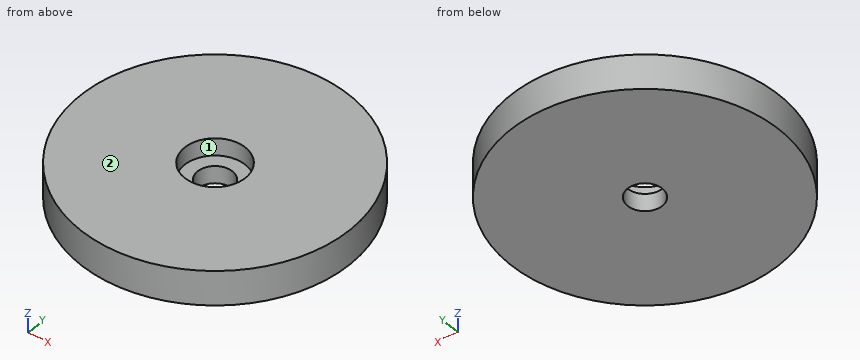
```python
from build123d import *

# Parameters (mm, degrees)
SKETCH_1_R          = 7.75
EXTRUDE_1_DEPTH     = 2
SKETCH_2_R          = 1
CUT_EXTRUDE_1_DEPTH = 12.141139978
SKETCH_2_3_R        = 1.75
SKETCH_2_3_R_2      = 1
CUT_EXTRUDE_2_DEPTH = 1


with BuildPart() as part:
    # 草图1 → 凸台-拉伸1 (new body)
    with BuildSketch(Plane.XY):
        Circle(SKETCH_1_R)
    extrude(amount=EXTRUDE_1_DEPTH)

    # 草图2 → 切除-拉伸1 (cut, through all)
    with BuildSketch(Plane.XY.offset(2)):
        Circle(SKETCH_2_R)
    extrude(amount=-CUT_EXTRUDE_1_DEPTH, mode=Mode.SUBTRACT)

    # 草图2<3> → 切除-拉伸2 (cut)
    with BuildSketch(Plane.XY.offset(2)):
        Circle(SKETCH_2_3_R)
        Circle(SKETCH_2_3_R_2, mode=Mode.SUBTRACT)
    extrude(amount=-CUT_EXTRUDE_2_DEPTH, mode=Mode.SUBTRACT)


solid = part.part
```
Here's how the part is built. I have some questions about the finished solid (model axes, mm). Face numbers are marked on the shaded views. A direction names the side the tool comes from. Coordinates: 2 decimals unless noted, no trailing zeros. Order: outer loops, then holes, each group sorted by start corner. A loop starts at its lowest first (then second) coordinate and runs counter-clockwise, first axis right, second up. Notation, with made-up numbers: (-13.5, -5) - (21.5, -5) arc R20 cw to (21.5, 21) - close; hole circle Ø11 at (-25, 61). An arc over 180 degrees is marked (long way). One line per question, with ' | ' between items. Start each with the question number.
1. Which directions (+Z, -Z, +X, -X, +Y, -Y) give clear straight access to the entire face, cutting with the end or side of a thin tool? Please do the marked faces 1 and 2.
2. If we section it at A-A (y = 0): Write out the boundary of the cut face in (x, z), and give its area (3 significant figures).
3. If we section it at D-D (z = 1.3): Write out the boundary of the cut face in (x, y).
4. Please list where these lines run through material, in increasing order: line 1 along Y through (x, z) = (0, 0.65); line 2 along X through (y, z) = (1.5, 1.35); line 3 along Y through (x, z) = (0, 1.6). Write a range as [from, to].
5. I'm going to push flat-ended pins straight in: pin 1 Ø1 at (x, z) = (-4.5, 0.5) entering from -Y; pin 2 Ø3 at (x, y) = (0, 0) entering from +Z; pin 3 Ø1 at (x, z) = (2.5, 1) entering from +Y. Where does each tip first touch, or does it pass through?
6. If we section it at C-C (z = 0.45): Write out the boundary of the cut face in (x, y).
Model answer:
1) face 1: +Z | face 2: +Z, +X, -X, +Y, -Y
2) outline: (-7.75, 0) - (-1, 0) - (-1, 1) - (-1.75, 1) - (-1.75, 2) - (-7.75, 2) - close; (1, 0) - (7.75, 0) - (7.75, 2) - (1.75, 2) - (1.75, 1) - (1, 1) - close | area: 25.5 mm²
3) outline: circle Ø15.5 at (0, 0); hole circle Ø3.5 at (0, 0)
4) line 1: y = [-7.75, -1], [1, 7.75] | line 2: x = [-7.6, -0.9], [0.9, 7.6] | line 3: y = [-7.75, -1.75], [1.75, 7.75]
5) pin 1: stops at y = -6.64 | pin 2: stops at z = 1 | pin 3: stops at y = 7.49
6) outline: circle Ø15.5 at (0, 0); hole circle Ø2 at (0, 0)
